```python
from build123d import *

# Parameters (mm, degrees)
SKETCH1_R           = 1.5
BOSS_EXTRUDE1_DEPTH = 4
SKETCH3_W           = 11.9
SKETCH3_H           = 17.9
BOSS_EXTRUDE2_DEPTH = 4
FILLET1_R           = 1
FILLET2_R           = 0.15


with BuildPart() as part:
    # Sketch1 → Boss-Extrude1 (new body)
    with BuildSketch(Plane.XY):
        with BuildLine():
            Line((3, 3), (3, -3))
            ThreePointArc((3, -3), (0, -6), (-3, -3))
            Line((-3, -3), (-3, 3))
            ThreePointArc((-3, 3), (0, 6), (3, 3))
        make_face()
        with Locations((0, 3)):
            Circle(SKETCH1_R, mode=Mode.SUBTRACT)
        with Locations((0, -3)):
            Circle(SKETCH1_R, mode=Mode.SUBTRACT)
    extrude(amount=BOSS_EXTRUDE1_DEPTH)

    # Sketch3 → Boss-Extrude2 (add)
    with BuildSketch(Plane.XY):
        Rectangle(SKETCH3_W, SKETCH3_H)
        with BuildLine():
            Line((3, 2.060806436), (3, 3))
            ThreePointArc((3, 3), (2.812460431, 4.044062414), (2.273289117, 4.957589484))
            ThreePointArc((2.273289117, 4.957589484), (3.195390382, 6.758191712), (4.663487388, 8.15))
            Line((4.663487388, 8.15), (-4.663487388, 8.15))
            ThreePointArc((-4.663487388, 8.15), (-3.195390382, 6.758191712), (-2.273289117, 4.957589484))
            ThreePointArc((-2.273289117, 4.957589484), (-2.812460431, 4.044062414), (-3, 3))
            Line((-3, 3), (-3, 2.060806436))
            ThreePointArc((-3, 2.060806436), (-3.713836261, 2.361122359), (-3.999178271, 3.081074995))
            ThreePointArc((-3.999178271, 3.081074995), (-4.282258248, 4.642222106), (-5.15, 5.970506272))
            Line((-5.15, 5.970506272), (-5.15, -5.970506272))
            ThreePointArc((-5.15, -5.970506272), (-4.282258248, -4.642222106), (-3.999178271, -3.081074995))
            ThreePointArc((-3.999178271, -3.081074995), (-3.713836261, -2.361122359), (-3, -2.060806436))
            Line((-3, -2.060806436), (-3, -3))
            ThreePointArc((-3, -3), (-2.812460431, -4.044062414), (-2.273289117, -4.957589484))
            ThreePointArc((-2.273289117, -4.957589484), (-3.195390382, -6.758191712), (-4.663487388, -8.15))
            Line((-4.663487388, -8.15), (4.663487388, -8.15))
            ThreePointArc((4.663487388, -8.15), (3.195390382, -6.758191712), (2.273289117, -4.957589484))
            ThreePointArc((2.273289117, -4.957589484), (2.812460431, -4.044062414), (3, -3))
            Line((3, -3), (3, -2.060806436))
            ThreePointArc((3, -2.060806436), (3.713836261, -2.361122359), (3.999178271, -3.081074995))
            ThreePointArc((3.999178271, -3.081074995), (4.282258248, -4.642222106), (5.15, -5.970506272))
            Line((5.15, -5.970506272), (5.15, 5.970506272))
            ThreePointArc((5.15, 5.970506272), (4.282258248, 4.642222106), (3.999178271, 3.081074995))
            ThreePointArc((3.999178271, 3.081074995), (3.713836261, 2.361122359), (3, 2.060806436))
        make_face(mode=Mode.SUBTRACT)
    extrude(amount=BOSS_EXTRUDE2_DEPTH)

    # Fillet1
    fillet1_edges = [part.edges().sort_by_distance(p)[0] for p in [
        (5.95, 8.95, 2),
        (-5.95, 8.95, 2),
        (-5.95, -8.95, 2),
        (5.95, -8.95, 2),
    ]]
    fillet(fillet1_edges, radius=FILLET1_R)

    # Fillet2
    fillet2_edges = [part.edges().sort_by_distance(p)[0] for p in [
        (-5.15, 5.970506272, 2),
        (-5.15, -5.970506272, 2),
        (-2.273289117, -4.957589484, 2),
        (-4.663487388, -8.15, 2),
        (4.663487388, -8.15, 2),
        (2.273289117, -4.957589484, 2),
        (5.15, -5.970506272, 2),
        (5.15, 5.970506272, 2),
        (2.273289117, 4.957589484, 2),
        (4.663487388, 8.15, 2),
        (-4.663487388, 8.15, 2),
        (-2.273289117, 4.957589484, 2),
    ]]
    fillet(fillet2_edges, radius=FILLET2_R)


solid = part.part
```
Can you work these out from the model? Positions are in its coordinate system, mm. A direction names the side the tool comes from. Coordinates: 2 decimals unless noted, no trailing zeros. Write each loop counter-clockwise with the first axis right and the second up, starting at its lowest first coordinate (ties: lowest second). Pieces come first, ordered by that corner, then holes. Notation, with made-up numbers: (0, -20.5) - (43, -20.5) arc R8 cw to (43, -15.5) - close; hole circle Ø11 at (85.5, 15.25). An arc over 180 degrees is marked (long way). Return JSON: item names as keys, results as strings.
Q1. I'm going to push a flat-ended pin straight in: pin 1 Ø2.5 at (x, y) = (0, -3) entering from -Z. Where does the tip first touch, or does it pass through?
Computed values:
{"pin 1": "passes through"}
Q2. If we section it at D-D (y = 3.75): Please give me the cut outline in (x, z), then the cut area to 3 significant figures.
Computed values:
{"outline": "(-5.95, 0) - (-5.15, 0) - (-5.15, 4) - (-5.95, 4) - close; (-4.04, 0) - (-1.3, 0) - (-1.3, 4) - (-4.04, 4) - close; (1.3, 0) - (4.04, 0) - (4.04, 4) - (1.3, 4) - close; (5.15, 0) - (5.95, 0) - (5.95, 4) - (5.15, 4) - close", "area": "28.3 mm2"}
Q3. If we section it at C-C (x = -1): Please give me the cut outline in (y, z).
Computed values:
{"outline": "(-8.95, 0) - (-8.15, 0) - (-8.15, 4) - (-8.95, 4) - close; (-5.83, 0) - (-4.12, 0) - (-4.12, 4) - (-5.83, 4) - close; (-1.88, 0) - (1.88, 0) - (1.88, 4) - (-1.88, 4) - close; (4.12, 0) - (5.83, 0) - (5.83, 4) - (4.12, 4) - close; (8.15, 0) - (8.95, 0) - (8.95, 4) - (8.15, 4) - close"}
Q4. Please list where these lines run through material, in increasing order: L1, parallel to X at y = -0.75, z = 0.7; L2, parallel to X at y = 3.5, z = 1.1; L3, parallel to X at y = 4.75, z = 0.45. Write a range as from..to.
Computed values:
{"L1": "x = -5.95..-5.15, -3..3, 5.15..5.95", "L2": "x = -5.95..-5.15, -4.01..-1.41, 1.41..4.01, 5.15..5.95", "L3": "x = -5.95..-5.15, -4.33..4.33, 5.15..5.95"}
Q5. On a 3-axis mill with a long thin cutter (end or side, diameter ignored), from which of +Z, -Z, +X, -X, +Y, -Y can I reach the whole of each face in a straight line? I mean faces 1 (the cylindrical face through (0, -6, 2)), 2 (the flat face through (-5.95, 0, 2)). Say none if no direction works.
Computed values:
{"face 1": "+Z, -Z", "face 2": "+Z, -Z, -X, +Y, -Y"}
Q6. If we section it at A-A (x = 3.5): Please give me the cut outline in (y, z), then the cut area to 3 significant figures.
Computed values:
{"outline": "(-8.95, 0) - (-8.15, 0) - (-8.15, 4) - (-8.95, 4) - close; (-7.13, 0) - (-2.2, 0) - (-2.2, 4) - (-7.13, 4) - close; (2.2, 0) - (7.13, 0) - (7.13, 4) - (2.2, 4) - close; (8.15, 0) - (8.95, 0) - (8.95, 4) - (8.15, 4) - close", "area": "45.9 mm2"}
Q7. If we section it at B-B (y = -7.25): Please give me the cut outline in (x, z).
Computed values:
{"outline": "(-5.95, 0) - (-3.61, 0) - (-3.61, 4) - (-5.95, 4) - close; (3.61, 0) - (5.95, 0) - (5.95, 4) - (3.61, 4) - close"}
Q8. Thinking about a two-plate mould opening in X: for faces 3 (the flat face through (0, -8.95, 2)), 4 (the cylindrical face through (-5.665, 8.649, 2.028)), 5 (the cylindrical face through (0, 6, 2)), which applies, +X half, -X half, draft (parallel to the pull), parting line (faces both ways), or undercut?
Computed values:
{"face 3": "draft", "face 4": "-X half", "face 5": "undercut"}
